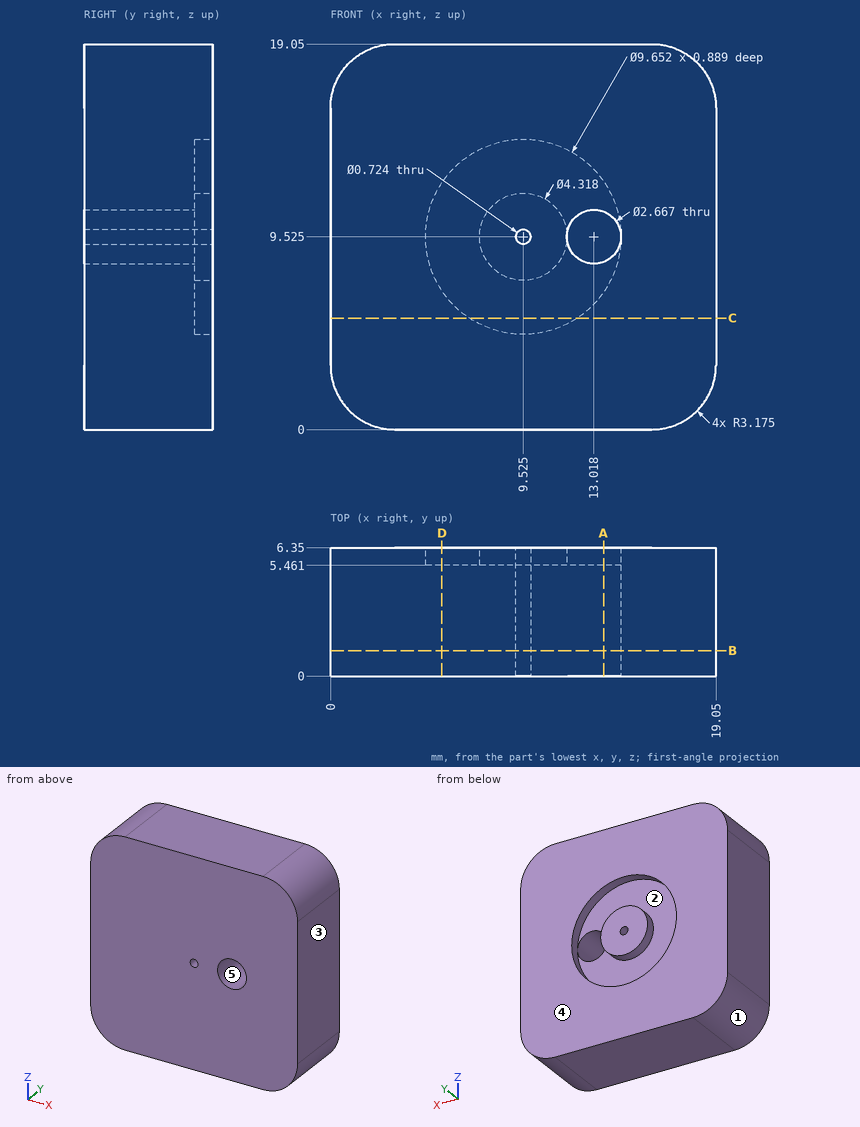
Could you check a few things on this drawing? It's one solid part, dimensions in mm from its lowest x, y, z. A direction names the side the tool comes from. Coordinates: 2 decimals unless noted, no trailing zeros. Order: outer loops, then holes, each group sorted by start corner. A loop starts at its lowest first (then second) coordinate and runs counter-clockwise, first axis right, second up. Notation, with made-up numbers: M 70,48.5 L 80,48.5 A31 ccw 80,72.5 Z; hole C -17,-28.75 d8. An arc over 180 degrees is marked long. Answer as a JSON object with one key per item and string values. Group by question number.
(1) Suppose I cut it at D-D, the plane x = 5.5. Please give me the cut outline in (y, z), then the cut area to 3 significant figures.
(2) Suppose I cut it at A-A, the plane x = 13.5. Please give me the cut outline in (y, z).
(3) Suppose I cut it at C-C, the plane z = 5.5. Please give me the cut outline in (x, y).
(4) Which directions (+Z, -Z, +X, -X, +Y, -Y) give clear straight access to the entire face, cutting with the end or side of a thin tool? Please do the marked faces 1 and 2.
(5) If we mould it in two halves opening along X, with no side actions, what happens to the marked faces 3, 4 and 5? For each: released by +X, released by -X, zero draft, split by the parting line, or undercut.
(6) Suppose I cut it at B-B, the plane y = 1.25. State how many separate pieces and enclosed holes the cut face has, then the cut area to 3 significant figures.
(7) I need wall thicknesses on probe 1 along Y at (x, z) = (5, 9.5); probe 2 along X at (y, z) = (5.5, 16); probe 3 along Z at (x, y) = (7.25, 5.75). Which ranges of each line are inside material? Lowest first, please.
Values found:
{
 "1": {"outline": "M 0,0 L 6.35,0 L 6.35,6.86 L 5.46,6.86 L 5.46,12.19 L 6.35,12.19 L 6.35,19.05 L 0,19.05 Z", "area": "116 mm^2"},
 "2": {"outline": "M 0,0 L 6.35,0 L 6.35,6.79 L 5.46,6.79 L 5.46,8.28 L 0,8.28 Z; M 0,10.77 L 5.46,10.77 L 5.46,12.26 L 6.35,12.26 L 6.35,19.05 L 0,19.05 Z"},
 "3": {"outline": "M 0,0 L 19.05,0 L 19.05,6.35 L 12.19,6.35 L 12.19,5.46 L 6.86,5.46 L 6.86,6.35 L 0,6.35 Z"},
 "4": {"face 1": "-Z, -X, +Y, -Y", "face 2": "+Y"},
 "5": {"face 3": "released by +X", "face 4": "zero draft", "face 5": "undercut"},
 "6": {"separate pieces": "1", "enclosed holes": "2", "area": "348 mm^2"},
 "7": {"probe 1": "y = 0 to 5.46", "probe 2": "x = 0 to 19.05", "probe 3": "z = 0 to 5.27, 13.78 to 19.05"}
}
